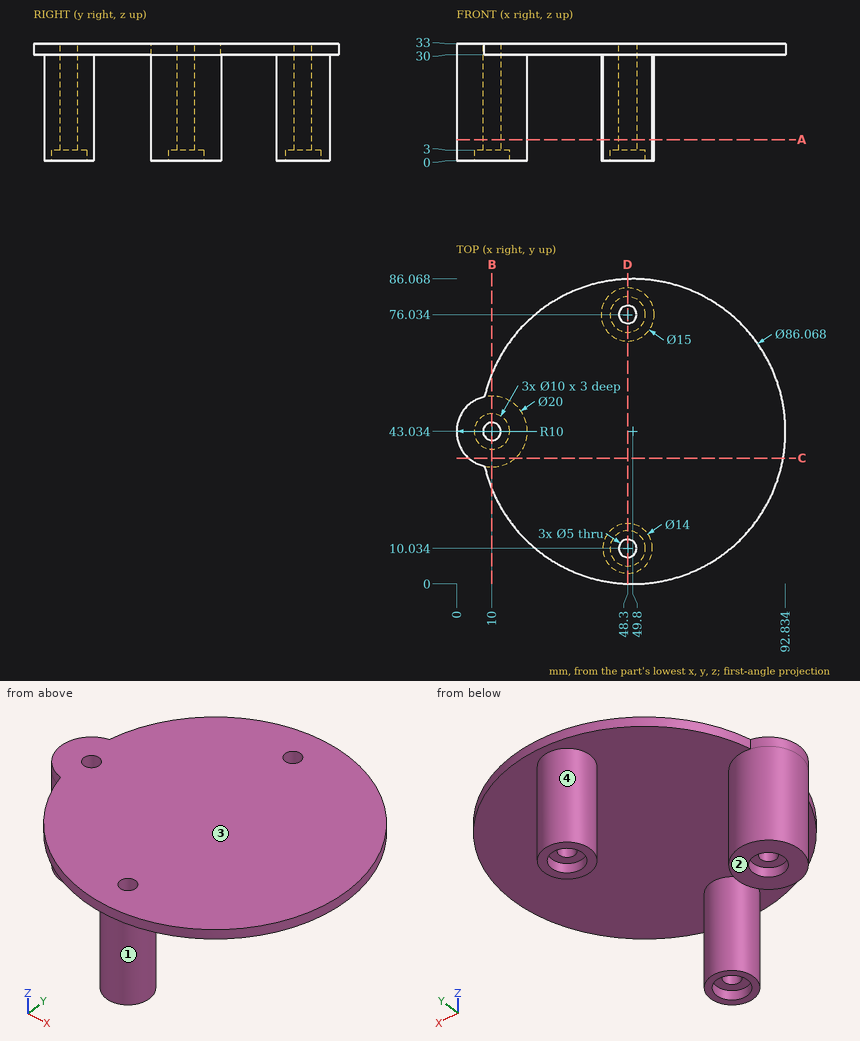
Could you check a few things on this drawing? It's one solid part, dimensions in mm from its lowest x, y, z. A direction names the side the tool comes from. Give positions to 0.01 mm unless a question says otherwise; leave off trailing zeros. Write each loop counter-clockwise with the first axis right and the second up, starting at its lowest first coordinate (ties: lowest second). Pieces come first, ordered by that corner, then holes. Notation, with made-up numbers: (6.5, 30) -> (35.5, 30) arc R19 cw to (35.5, 67) -> close; hole circle Ø3 at (19, 77). An arc over 180 degrees is marked (long way). Answer as a JSON object with one key per item and string values.
Q1. Suppose I cut it at B-B on x = 10. Write out the boundary of the cut face in (y, z), then the cut area to 3 significant figures.
Taken from the geometry:
{"outline": "(26.67, 30) -> (33.03, 30) -> (33.03, 0) -> (38.03, 0) -> (38.03, 3) -> (40.53, 3) -> (40.53, 33) -> (26.67, 33) -> close; (45.53, 3) -> (48.03, 3) -> (48.03, 0) -> (53.03, 0) -> (53.03, 30) -> (59.4, 30) -> (59.4, 33) -> (45.53, 33) -> close", "area": "518 mm²"}
Q2. Suppose I cut it at A-A on z = 6. Write out the boundary of the cut face in (x, y).
Taken from the geometry:
{"outline": "circle Ø20 at (10, 43.03); circle Ø15 at (48.3, 76.03); circle Ø14 at (48.3, 10.03); hole circle Ø5 at (10, 43.03); hole circle Ø5 at (48.3, 10.03); hole circle Ø5 at (48.3, 76.03)"}
Q3. Suppose I cut it at D-D on x = 48.3. Write out the boundary of the cut face in (y, z).
Taken from the geometry:
{"outline": "(0.03, 30) -> (3.03, 30) -> (3.03, 0) -> (5.03, 0) -> (5.03, 3) -> (7.53, 3) -> (7.53, 33) -> (0.03, 33) -> close; (12.53, 3) -> (15.03, 3) -> (15.03, 0) -> (17.03, 0) -> (17.03, 30) -> (68.53, 30) -> (68.53, 0) -> (71.03, 0) -> (71.03, 3) -> (73.53, 3) -> (73.53, 33) -> (12.53, 33) -> close; (78.53, 3) -> (81.03, 3) -> (81.03, 0) -> (83.53, 0) -> (83.53, 30) -> (86.04, 30) -> (86.04, 33) -> (78.53, 33) -> close"}
Q4. Will these pins go through, and if not, where does the flat tip stop? pin 1 Ø12 at (x, z) = (16.5, 23.5) entering from -Y; pin 2 Ø1 at (x, y) = (79, 60.5) entering from -Z; pin 3 Ø5 at (x, y) = (50, 76) entering from -Z.
Taken from the geometry:
{"pin 1": "stops at y = 33.05", "pin 2": "stops at z = 30", "pin 3": "stops at z = 3"}
Q5. We'd pull the mould along Y, two halves only. Please class the marked faces 1 and 2: released by +Y, released by -Y, zero draft, split by the parting line, or undercut.
Taken from the geometry:
{"face 1": "undercut", "face 2": "zero draft"}
Q6. Suppose I cut it at C-C on y = 35.5. Write out the boundary of the cut face in (x, z).
Taken from the geometry:
{"outline": "(3.42, 0) -> (16.58, 0) -> (16.58, 30) -> (92.17, 30) -> (92.17, 33) -> (3.42, 33) -> close"}
Q7. Which directions (+Z, -Z, +X, -X, +Y, -Y) give clear straight access to the entire face, cutting with the end or side of a thin tool? Please do the marked faces 3 and 4.
Taken from the geometry:
{"face 3": "+Z, +X, -X, +Y, -Y", "face 4": "-Z"}
Q8. Please list where these lines run through material, in increasing order: L1, parallel to Y at x = 48.3, z = 1.7; L2, parallel to Y at x = 48.3, z = 12.5; L3, parallel to Y at x = 10, z = 2.
Taken from the geometry:
{"L1": "y = 3.03 to 5.03, 15.03 to 17.03, 68.53 to 71.03, 81.03 to 83.53", "L2": "y = 3.03 to 7.53, 12.53 to 17.03, 68.53 to 73.53, 78.53 to 83.53", "L3": "y = 33.03 to 38.03, 48.03 to 53.03"}
